from build123d import *

# Parameters (mm, degrees)
BOSS_EXTRUDE1_DEPTH          = 1.25
BOSS_EXTRUDE8_START          = -8
BOSS_EXTRUDE8_DEPTH          = 16
CHAMFER2_SIZE2               = 3
CHAMFER2_SIZE                = 1.25
CHAMFER3_SIZE2               = 3
CHAMFER3_SIZE                = 1.25
BOSS_EXTRUDE9_DEPTH          = 1.25
BOSS_EXTRUDE10_DEPTH         = 1.25
CUT_EXTRUDE1_REACH           = 59.082
SKETCH6_R                    = 0.5
SCHIZZO1_R                   = 4
SCHIZZO1_R_2                 = 3
ESTRUSIONE_ESTRUSIONE1_DEPTH = 2.1
RACCORDO1_R                  = 0.45


with BuildPart() as part:
    # Sketch1 → Boss-Extrude1 (new body)
    with BuildSketch(Plane(origin=(0, 0, 0), x_dir=(1, 0, 0), z_dir=(0, 1, 0))):
        with BuildLine():
            Line((-50, 0), (-2.082988952, 21.95833302))
            ThreePointArc((-2.082988952, 21.95833302), (0, 22.412878475), (2.082988952, 21.95833302))
            Line((2.082988952, 21.95833302), (50, 0))
            Line((50, 0), (20, 0))
            Line((20, 0), (0.753370804, 22.049783791))
            ThreePointArc((0.753370804, 22.049783791), (0, 22.392187842), (-0.753370804, 22.049783791))
            Line((-0.753370804, 22.049783791), (-20, 0))
            Line((-20, 0), (-50, 0))
        make_face()
    extrude(amount=BOSS_EXTRUDE1_DEPTH)


with BuildPart() as body_2:
    # Body-Move/Copy1: copy of part
    add(part.part.moved(Location((0, 14.75, 0))))


with BuildPart() as part_1:
    add(part.part)

    add(body_2.part)  # Boss-Extrude8 merges body 2
    # Sketch3 → Boss-Extrude8 (add)
    with BuildSketch(Plane(origin=(0, 8, 0), x_dir=(1, 0, 0), z_dir=(0, 1, 0)).offset(BOSS_EXTRUDE8_START)):
        with BuildLine():
            Line((19.431879943, -1.25), (0, 21.012015184))
            Line((0, 21.012015184), (-19.431879943, -1.25))
            Line((-19.431879943, -1.25), (-50, -1.25))
            Line((-50, -1.25), (-50, 0))
            Line((-50, 0), (-20, 0))
            Line((-20, 0), (-0.753370804, 22.049783791))
            ThreePointArc((-0.753370804, 22.049783791), (0, 22.392187842), (0.753370804, 22.049783791))
            Line((0.753370804, 22.049783791), (20, 0))
            Line((20, 0), (50, 0))
            Line((50, 0), (50, -1.25))
            Line((50, -1.25), (19.431879943, -1.25))
        make_face()
    extrude(amount=BOSS_EXTRUDE8_DEPTH)

    # Chamfer2
    chamfer2_edges = [part_1.edges().sort_by_distance(p)[0] for p in [
        (50, 8, 1.25),
    ]]
    chamfer2_side = [part_1.faces().sort_by_distance(p)[0] for p in [
        (50, 8, 1.225),
    ]]
    chamfer(chamfer2_edges, length=CHAMFER2_SIZE - 0.0001, length2=CHAMFER2_SIZE2 - 0.0001, reference=chamfer2_side[0])  # a hair under: the kernel refuses the full size

    # Chamfer3
    chamfer3_edges = [part_1.edges().sort_by_distance(p)[0] for p in [
        (-50, 8, 1.25),
    ]]
    chamfer3_side = [part_1.faces().sort_by_distance(p)[0] for p in [
        (-50, 8, 1.225),
    ]]
    chamfer(chamfer3_edges, length=CHAMFER3_SIZE - 0.0001, length2=CHAMFER3_SIZE2 - 0.0001, reference=chamfer3_side[0])  # a hair under: the kernel refuses the full size

    # Sketch4 → Boss-Extrude9 (add)
    with BuildSketch(Plane(origin=(0, 16, 0), x_dir=(1, 0, 0), z_dir=(0, 1, 0))):
        Polygon((-19.431879943, -1.25), (0, 21.012015184), (19.431879943, -1.25), align=None)
    boss_extrude9 = extrude(amount=-BOSS_EXTRUDE9_DEPTH)

    # Mirror1: Boss-Extrude9 across plane
    add(boss_extrude9.mirror(Plane.ZX.offset(8)))

    # Sketch5 → Boss-Extrude10 (add)
    with BuildSketch(Plane.XZ):
        with BuildLine():
            Line((-7.5, 1.25), (7.5, 1.25))
            Line((7.5, 1.25), (1.499675711, 8.050367528))
            ThreePointArc((1.499675711, 8.050367528), (0, 8.727124254), (-1.499675711, 8.050367528))
            Line((-1.499675711, 8.050367528), (-7.5, 1.25))
        make_face()
    boss_extrude10 = extrude(amount=-BOSS_EXTRUDE10_DEPTH)

    # Mirror2: Boss-Extrude10 across plane
    add(boss_extrude10.mirror(Plane.ZX.offset(8)))

    # Sketch6 → Cut-Extrude1 (cut, up to next)
    with BuildSketch(Plane(origin=(0, 0, 0), x_dir=(-1, 0, 0), z_dir=(0, -1, 0)), mode=Mode.PRIVATE) as cut_extrude1_sk1:
        with Locations(Location((0, -5.727124254, 0), (0, 0, 90))):
            Circle(SKETCH6_R)
    cut_extrude1_tool1 = extrude(cut_extrude1_sk1.sketch, amount=-CUT_EXTRUDE1_REACH, mode=Mode.PRIVATE) & part_1.part
    add(cut_extrude1_tool1.solids().sort_by_distance((0, 0, 5.727124))[0], mode=Mode.SUBTRACT)
    add(cut_extrude1_tool1.solids().sort_by_distance((0, 0, 5.727124))[1], mode=Mode.SUBTRACT)

    # Schizzo1 → Estrusione-Estrusione1 (add)
    with BuildSketch(Plane(origin=(0, 16, 0), x_dir=(1, 0, 0), z_dir=(0, 1, 0))):
        with Locations(Location((0, 17.912878475, 0), (0, 0, 270))):
            Circle(SCHIZZO1_R)
        with Locations(Location((0, 17.912878475, 0), (0, 0, 270))):
            Circle(SCHIZZO1_R_2, mode=Mode.SUBTRACT)
    extrude(amount=ESTRUSIONE_ESTRUSIONE1_DEPTH)

    # Raccordo1
    raccordo1_edges = [part_1.edges().sort_by_distance(p)[0] for p in [
        (0, 18.1, -21.912878475),
        (0, 16, -21.912878475),
        (0, 18.1, -20.912878475),
    ]]
    fillet(raccordo1_edges, radius=RACCORDO1_R)


solid = part_1.part
The model under review builds one solid part; all positions refer to its coordinate system, in mm. A direction names the side the tool comes from. Round coordinates to 2 decimals unless told otherwise and drop trailing zeros. Loops run counter-clockwise (first coordinate to the right, second up) from the corner with the lowest first, then second, coordinate; pieces in that order, holes last. Notation, with made-up numbers: M 31.5,61.5 L 61.5,61.5 A4 ccw 61.5,68.5 Z; hole C 41,29.25 d9. An arc over 180 degrees is marked long. Answer as a JSON object with one key per item and string values.
Item 1: We need section D-D, the plane x = -15.5. State the section outline as (y, z) points, and give its area (3 significant figures).
Check sheet entries:
{"outline": "M 0,-15.81 L 1.25,-15.81 L 1.25,-5.16 L 14.75,-5.16 L 14.75,-15.81 L 16,-15.81 L 16,1.25 L 14.75,1.25 L 14.75,-3.25 L 1.25,-3.25 L 1.25,1.25 L 0,1.25 Z", "area": "68.3 mm2"}
Item 2: Clearance check with flat-ended pins moving along their axes: P1, Ø6.5, axis at x = -0.5, z = -19, coming from the +Y side; P2, Ø10, axis at x = -24.5, z = -3, coming from the +Y side; P3, Ø10, axis at x = -14, y = 11.5, coming from the -Z side; P4, Ø2, axis at y = 5.5, z = -17, coming from the +X side. State where each tip first meets the part, or that it passes through.
Check sheet entries:
{"P1": "y = 18.1", "P2": "y = 16", "P3": "z = -18.24", "P4": "x = 6.03"}
Item 3: The part is to be moulded in two halves that separate along Y. For faces 5 (the face through (9.85, 7.91, -9.73)), 6 (the face through (-9.58, 7.906, -10.037)), 7 (the face through (0, 16, -18)), 8 (the face through (4.542, 15.384, 4.603)), say which applies: +Y half, -Y half, draft (parallel to the pull), parting line (faces both ways), or undercut.
Check sheet entries:
{"face 5": "undercut", "face 6": "undercut", "face 7": "+Y half", "face 8": "draft"}
Item 4: We need section C-C, the plane x = -34. State the section outline as (y, z) points, and give its area (3 significant figures).
Check sheet entries:
{"outline": "M 0,-7.33 L 1.25,-7.33 L 1.25,0 L 14.75,0 L 14.75,-7.33 L 16,-7.33 L 16,1.25 L 0,1.25 Z", "area": "38.3 mm2"}
Item 5: Tool access review of faces 1 (the face through (-7.2, 1.25, -15.4)), 2 (the face through (-1.532, 17.042, -14.218)), 3 (the face through (10.24, 7.91, -11.18)), 4 (the face through (-31, 8, 1.25)): name each direction out of +Z, -Z, +X, -X, +Y, -Y from which nothing blocks a thin tool from reaching the whole face with its end or side.
Check sheet entries:
{"face 1": "-Z", "face 2": "+Y", "face 3": "-Z, +X", "face 4": "+Z, -X, +Y, -Y"}
Item 6: We need section B-B, the plane z = -12. State the section outline as (x, y) points, and give its area (3 significant figures).
Check sheet entries:
{"outline": "M -23.81,0 L 23.81,0 L 23.81,1.25 L 9.53,1.25 L 9.53,14.75 L 23.81,14.75 L 23.81,16 L -23.81,16 L -23.81,14.75 L -9.53,14.75 L -9.53,1.25 L -23.81,1.25 Z; hole M -7.87,1.25 L 7.87,1.25 L 7.87,14.75 L -7.87,14.75 Z", "area": "164 mm2"}
Item 7: For line 1 along Y through (x, z) = (15, -8); line 2 along Z through (x, y) = (-35.5, 11); line 3 along X through (y, z) = (5, -0.5), list the stretches that pass through material, from the lowest coordinate up.
Check sheet entries:
{"line 1": "0 to 1.25, 14.75 to 16", "line 2": "0 to 1.25", "line 3": "-19.56 to -17.9, 17.9 to 19.56"}
